```python
from build123d import *

# Parameters (mm, degrees)
F1_DEPTH = 0.5
F4_ANGLE = -45


with BuildPart() as f1:
    # F0 (on Right) → F1 (new body)
    with BuildSketch(Plane.YZ):
        Polygon((-20, 0), (-30, -18), (0, -18), (10, 0), (0, 0), align=None)
    extrude(amount=F1_DEPTH)


with BuildPart() as f1_1:
    # F3: moved
    add(f1.part.moved(Location((-0.5, 30, -77))))


with BuildPart() as f1_2:
    # F4: moved
    add(f1_1.part.rotate(Axis((-0.25, 0, -95), (-1, 0, 0)), F4_ANGLE))


with BuildPart() as f1_3:
    # F5: moved
    add(f1_2.part.moved(Location((0, -3, 0))))


solid = f1_3.part
```
Part model, mm, in its own coordinate system. Coordinates: 2 decimals unless noted, no trailing zeros. Order: outer loops, then holes, each group sorted by start corner. A loop starts at its lowest first (then second) coordinate and runs counter-clockwise, first axis right, second up. Notation, with made-up numbers: (-13, 25.25) -> (40, 25.25) arc R23 ccw to (40, 60.25) -> close; hole circle Ø7 at (85.25, 12.25). An arc over 180 degrees is marked (long way). Put each result on its own line as item: value. Start each with the question number.
(1) Band-saw the part on B-B (y = 16.25). Give the cut face in (x, z), then the cut area to 3 significant figures.
(2) Probe line 1 along Y through (x, z) = (-0.05, -59.5); line 2 along Y through (x, z) = (-0.05, -64); line 3 along Z through (x, y) = (-0.4, 3). List the from-to ranges inside material, lowest first. Write a range as [from, to].
(3) Band-saw the part on A-A (x = -0.35). Give the cut face in (y, z), then the cut area to 3 significant figures.
Determined:
1. outline: (-0.5, -75.75) -> (0, -75.75) -> (0, -66.92) -> (-0.5, -66.92) -> close
1. area: 4.42 mm²
2. line 1: y = [7.04, 14.13]
2. line 2: y = [2.54, 15.42]
2. line 3: z = [-89, -63.54]
3. outline: (-8.66, -75.2) -> (-3, -95) -> (18.21, -73.79) -> (12.56, -53.99) -> close
3. area: 540 mm²
